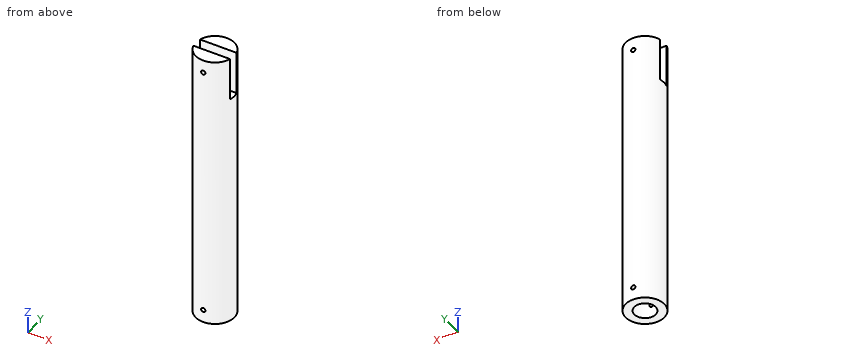
```python
from build123d import *

# Parameters (mm, degrees)
SZKIC1_R                    = 4.5
DODANIE_WYCI_GNI_CIE1_DEPTH = 65
WYTNIJ_WYCI_GNI_CIE1_START  = -10
WYTNIJ_WYCI_GNI_CIE1_DEPTH  = 10
SZKIC3_R                    = 2.5
WYTNIJ_WYCI_GNI_CIE3_DEPTH  = 6
SZKIC4_R                    = 0.5
WYTNIJ_WYCI_GNI_CIE4_DEPTH  = 66.310795432


with BuildPart() as part:
    # Szkic1 → Dodanie-wyciągnięcie1 (new body)
    with BuildSketch(Plane.XY):
        Circle(SZKIC1_R)
    extrude(amount=DODANIE_WYCI_GNI_CIE1_DEPTH)

    # Szkic2 → Wytnij-wyciągnięcie1 (cut)
    with BuildSketch(Plane.XY.offset(65).offset(WYTNIJ_WYCI_GNI_CIE1_START)):
        with BuildLine():
            Line((-4.322904116, 1.25), (4.322904116, 1.25))
            ThreePointArc((4.322904116, 1.25), (4.5, 0), (4.322904116, -1.25))
            Line((4.322904116, -1.25), (-4.322904116, -1.25))
            ThreePointArc((-4.322904116, -1.25), (-4.5, 0), (-4.322904116, 1.25))
        make_face()
    extrude(amount=WYTNIJ_WYCI_GNI_CIE1_DEPTH, mode=Mode.SUBTRACT)

    # Szkic3 → Wytnij-wyciągnięcie3 (cut)
    with BuildSketch(Plane(origin=(0, 0, 0), x_dir=(-1, 0, 0), z_dir=(0, 0, -1))):
        Circle(SZKIC3_R)
    extrude(amount=-WYTNIJ_WYCI_GNI_CIE3_DEPTH, mode=Mode.SUBTRACT)

    # Szkic4 → Wytnij-wyciągnięcie4 (cut, symmetric)
    with BuildSketch(Plane(origin=(0, 0, 0), x_dir=(1, 0, 0), z_dir=(0, 1, 0))):
        with Locations(Location((0, -3, 0), (0, 0, 90))):
            Circle(SZKIC4_R)
    wytnij_wyci_gni_cie4 = extrude(amount=WYTNIJ_WYCI_GNI_CIE4_DEPTH, both=True, mode=Mode.SUBTRACT)

    # Lustro1: Wytnij-wyciągnięcie4 across plane
    add(wytnij_wyci_gni_cie4.mirror(Plane(origin=(0, 0, 32.5), x_dir=(1, 0, 0), z_dir=(0, 0, -1))), mode=Mode.SUBTRACT)


solid = part.part
```
Build history of the part. All positions in model axes, mm. Give positions to 0.01 mm unless a question says otherwise; leave off trailing zeros. Order: outer loops, then holes, each group sorted by start corner. A loop starts at its lowest first (then second) coordinate and runs counter-clockwise, first axis right, second up. Notation, with made-up numbers: M -35.75,-20.5 L 7.25,-20.5 A22 cw 7.25,1.5 Z; hole C -9,60.25 d10. An arc over 180 degrees is marked long. Write item = value, one per line. Start each with the question number.
(1) Slice it at D-D on z = 30.5. Write the cut outline in (x, y), plus the area to 3 significant figures.
(2) Slice it at B-B on z = 56.5. Write the cut outline in (x, y), plus the area to 3 significant figures.
(3) Slice it at C-C on y = -3.5. Write the cut outline in (x, z), plus the area to 3 significant figures.
(4) Probe L1, parallel to Y at x = 0, z = 4.75; L2, parallel to Y at x = -1.25, z = 55.5; L3, parallel to X at y = 3.75, z = 42. List the from-to ranges inside material, lowest first. Write a range as [from, to].
(5) Slice it at A-A on y = 0. Write the cut outline in (x, z), plus the area to 3 significant figures.
(6) Pin check, flat tips, straight feed: pin 1 Ø2.5 at (x, y) = (0.5, 0.5) entering from -Z; pin 2 Ø1.5 at (y, z) = (3, 9.5) entering from -X. Stop position of each tip, or through.
Responses:
q1.outline = C 0,0 d9
q1.area = 63.6 mm2
q2.outline = M -4.32,-1.25 A4.5 ccw 4.32,-1.25 Z; M -4.32,1.25 L 4.32,1.25 A4.5 ccw Z
q2.area = 41.4 mm2
q3.outline = M -2.83,0 L 2.83,0 L 2.83,65 L -2.83,65 Z; hole C 0,3 d1; hole C 0,62 d1
q3.area = 366 mm2
q4.L1 = [-4.5, -2.5], [2.5, 4.5]
q4.L2 = [-4.32, -1.25], [1.25, 4.32]
q4.L3 = [-2.49, 2.49]
q5.outline = M -4.5,0 L -2.5,0 L -2.5,6 L 2.5,6 L 2.5,0 L 4.5,0 L 4.5,55 L -4.5,55 Z
q5.area = 465 mm2
q6.pin_1 = 6
q6.pin_2 = -3.9
